```python
from build123d import *

# Parameters (mm, degrees)
F0_R          = 71.5623861555
F1_DEPTH      = 12.7
F3_R          = 41.9736648942
F4_DEPTH      = 12.7
F4_TAPER      = 45
F5_R          = 15.5695486485
F6_DEPTH      = 25.4
F6_DEPTH_BACK = 25.4
F7_R          = 5.5767629642
F8_DEPTH      = 25.4
F9_R          = 5.08
F10_T         = -2.54


with BuildPart() as f1:
    # F0 (on Front) → F1 (new body)
    with BuildSketch(Plane.XZ):
        Circle(F0_R)
    extrude(amount=F1_DEPTH)

    # F3 (on offset) → F4 (join)
    with BuildSketch(Plane.XZ.offset(12.7)):
        Circle(F3_R)
    extrude(amount=F4_DEPTH, taper=F4_TAPER)

    # F5 (on offset) → F6 (cut, two sides)
    with BuildSketch(Plane.XZ.offset(12.7)) as f6_sk:
        Circle(F5_R)
    extrude(amount=-F6_DEPTH, mode=Mode.SUBTRACT)
    extrude(f6_sk.sketch, amount=F6_DEPTH_BACK, mode=Mode.SUBTRACT)

    # F7 (on Front) → F8 (cut)
    with BuildSketch(Plane.XZ):
        with Locations((0, 55.3915388882)):
            Circle(F7_R)
        with Locations((-39.1677327682, 39.1677327682)):
            Circle(F7_R)
        with Locations((-55.3915388882, 0)):
            Circle(F7_R)
        with Locations((-39.1677327682, -39.1677327682)):
            Circle(F7_R)
        with Locations((0, -55.3915388882)):
            Circle(F7_R)
        with Locations((39.1677327682, -39.1677327682)):
            Circle(F7_R)
        with Locations((55.3915388882, 0)):
            Circle(F7_R)
        with Locations((39.1677327682, 39.1677327682)):
            Circle(F7_R)
    extrude(amount=F8_DEPTH, mode=Mode.SUBTRACT)

    # F9
    f9_edges = [f1.edges().sort_by_distance(p)[0] for p in [
        (-71.562386, -12.7, 0),
        (-41.973665, -12.7, 0),
        (-29.273665, -25.4, 0),
    ]]
    fillet(f9_edges, radius=F9_R)

    # F10
    f10_openings = [f1.faces().sort_by_distance(p)[0] for p in [
        (-69.538296, 0, 0),
    ]]
    offset(amount=F10_T, openings=f10_openings)


solid = f1.part
```
Work out the finished part from the listing and answer in its coordinate system (mm). A direction names the side the tool comes from. Coordinates: 2 decimals unless noted, no trailing zeros.
1) Flat-ended cylindrical pins translate along their axes: pin 1 (4 mm diameter, centred on x = 45.5, z = -53, fed in from -Y); pin 2 (4 mm diameter, centred on x = 53.5, y = -11, fed in from -Z); pin 3 (14.5 mm diameter, centred on x = 39.17, z = 39.17, fed in from -Y); pin 4 (6 mm diameter, centred on x = 15.5, z = 1, fed in from +Y). Find the tip coordinate at first contact, or state that the pin passes through.
Results:
pin 1: stops at y = -12.51
pin 2: stops at z = -48.56
pin 3: stops at y = -12.7
pin 4: stops at y = 0
2) Consider probe 1 along Z at (x, y) = (-48, -3); probe 2 along X at (y, z) = (-13.75, 8.5); probe 3 along X at (y, z) = (-19, -2). Determine where each line is inside the solid, lowest interval first.
Results:
probe 1: z = -53.08 to -49.6, -3.35 to 3.35, 49.6 to 53.08
probe 2: x = -40.09 to -36.35, -15.99 to -13.04, 13.04 to 15.99, 36.35 to 40.09
probe 3: x = -35.62 to -32.02, -18 to -15.44, 15.44 to 18, 32.02 to 35.62
3) Section A-A (x = 0) is taken. Give the number of separate pieces and of enclosed holes in the cut face, plus the area to 3 significant figures.
Results:
separate pieces: 4
enclosed holes: 0
area: 515 mm2
4) For a pull along Z with two mould halves and no side action, classify faces 1 (the conical face through (-4.07, -23.44, 30.97)), 2 (the flat face through (14, -12.7, -43)), 3 (the cylindrical face through (46.9, -5, -36.7)) as +Z half, -Z half, draft (parallel to the pull), parting line (faces both ways), or undercut.
Results:
face 1: parting line
face 2: draft
face 3: undercut
5) For faces 4 (the flat face through (-37, 0, 45)), 5 (the cylindrical face through (-31.67, -5.01, -42.28)), determine the directions among +Z, -Z, +X, -X, +Y, -Y from which every point of the face is accessible in a straight line to the end or side of a thin tool.
Results:
face 4: +Z, -Z, +X, -X, +Y
face 5: +Y
